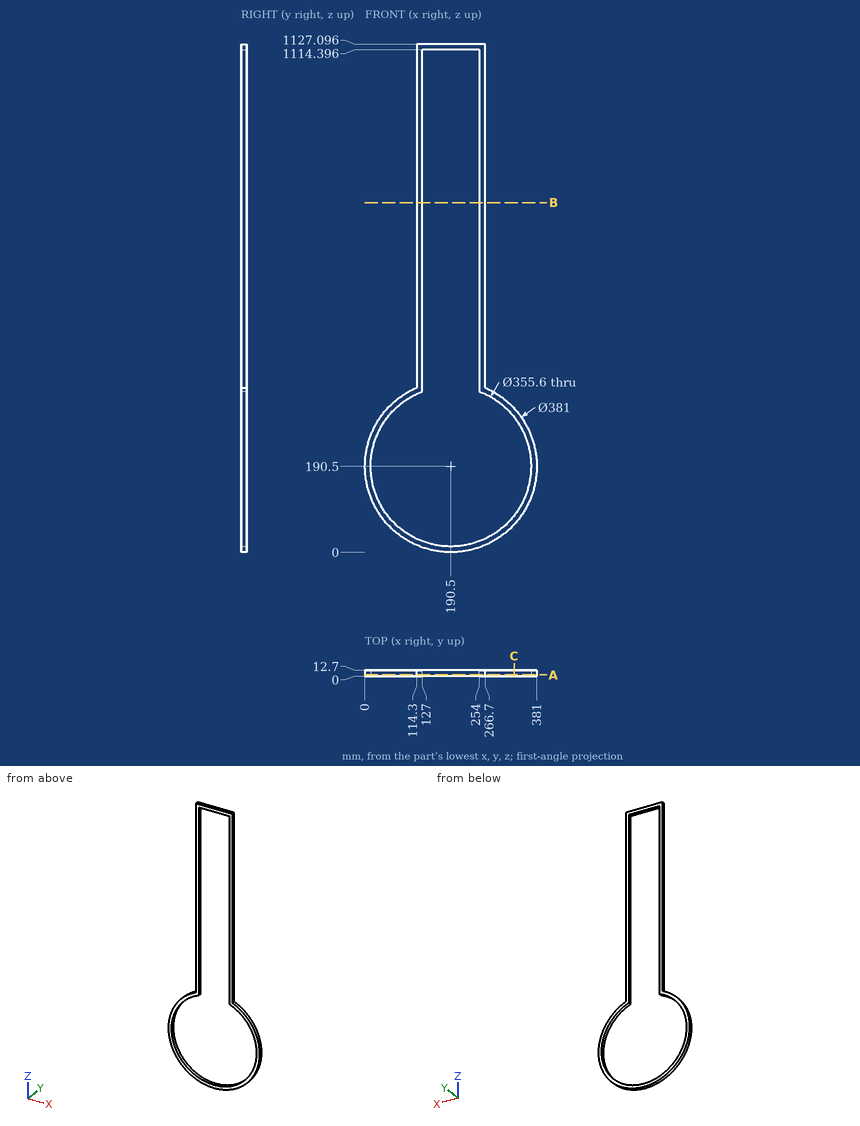
Study the drawing (mm; zero at the part's minimum x, y, z) and answer. Give positions to 0.01 mm unless a question says otherwise; leave off trailing zeros. Write each loop counter-clockwise with the first axis right and the second up, starting at its lowest first coordinate (ties: lowest second). Pieces come first, ordered by that corner, then holes.
(1) The part is cut by section C-C on x = 331. Write down the section's boundary in (y, z), plus the area to 3 significant figures.
Final values:
outline: (0, 61.85) - (12.7, 61.85) - (12.7, 81.54) - (0, 81.54) - close; (0, 299.46) - (12.7, 299.46) - (12.7, 319.15) - (0, 319.15) - close
area: 500 mm2
(2) The part is cut by section B-B on z = 775.5. Write down the section's boundary in (x, y).
Final values:
outline: (114.3, 0) - (127, 0) - (127, 12.7) - (114.3, 12.7) - close; (254, 0) - (266.7, 0) - (266.7, 12.7) - (254, 12.7) - close
(3) The part is cut by section A-A on y = 2.5. Write down the section's boundary in (x, z).
Final values:
outline: (114.3, 365.1) arc R190.5 ccw (long way) to (266.7, 365.1) - (266.7, 1127.1) - (114.3, 1127.1) - close; hole (127, 356.57) arc R177.8 ccw (long way) to (254, 356.57) - (254, 1114.4) - (127, 1114.4) - close
(4) Straight lines are drawn through the part: line 1 (X direction, y = 4.5, z = 692); line 2 (Z direction, x = 257.5, y = 10); line 3 (Z direction, x = 48, y = 6.75). For each, find the intervals that lie inside material, in ascending order.
Final values:
line 1: x = 114.3 to 127, 254 to 266.7
line 2: z = 12.17 to 25.81, 355.19 to 1127.1
line 3: z = 64.07 to 84.17, 296.83 to 316.93
(5) Flat-ended cylindrical pins translate along their axes: pin 1 Ø4 at (y, z) = (9, 565) entering from -X; pin 2 Ø5 at (y, z) = (8.5, 355.5) entering from -X; pin 3 Ø6.5 at (x, y) = (204.5, 6.5) entering from -Z. Find the tip coordinate at first contact, or state that the pin passes through.
Final values:
pin 1: stops at x = 114.3
pin 2: stops at x = 91.08
pin 3: stops at z = 0.3
